Job drawing, mm, ordinate dimensions from the low corner. One solid piece. Round coordinates to 2 decimals unless told otherwise and drop trailing zeros. Loops run counter-clockwise (first coordinate to the right, second up) from the corner with the lowest first, then second, coordinate; pieces in that order, holes last.
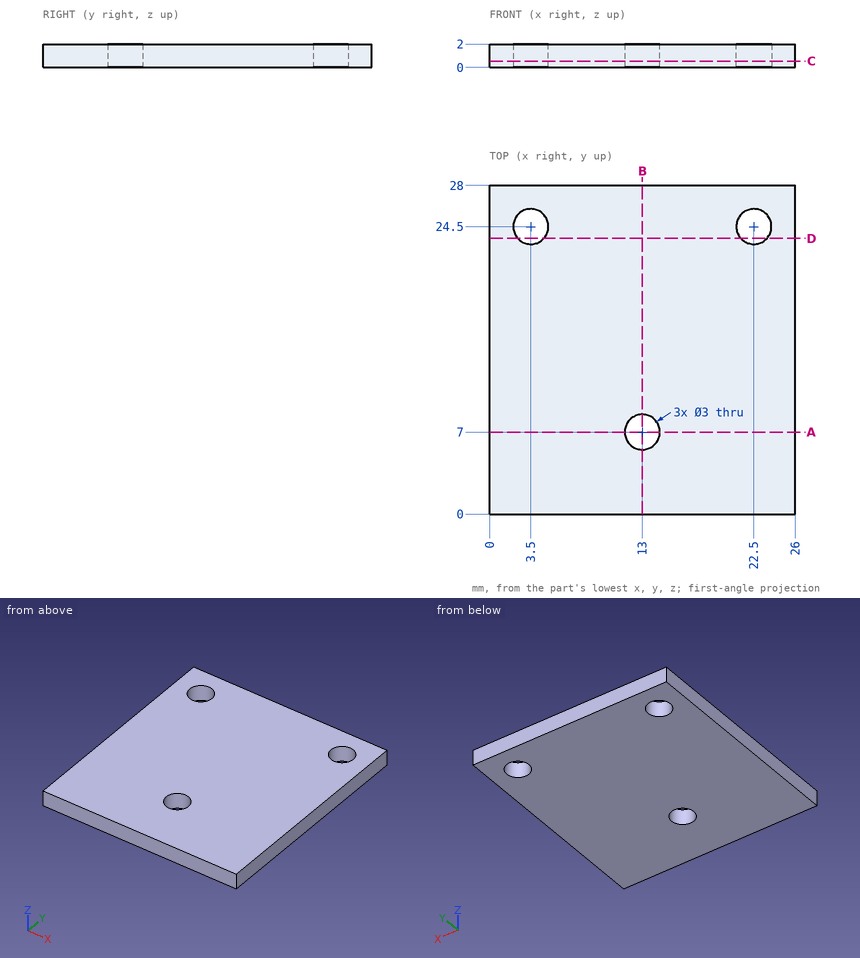
Item 1: Cut at A-A, the plane y = 7. Give the cut face in (x, z), plus the area to 3 significant figures.
Answers follow:
outline: (0, 0) - (11.5, 0) - (11.5, 2) - (0, 2) - close; (14.5, 0) - (26, 0) - (26, 2) - (14.5, 2) - close
area: 46.0 mm2
Item 2: Cut at D-D, the plane y = 23.5. Give the cut face in (x, z), plus the area to 3 significant figures.
Answers follow:
outline: (0, 0) - (2.38, 0) - (2.38, 2) - (0, 2) - close; (4.62, 0) - (21.38, 0) - (21.38, 2) - (4.62, 2) - close; (23.62, 0) - (26, 0) - (26, 2) - (23.62, 2) - close
area: 43.1 mm2
Item 3: Cut at C-C, the plane z = 0.55. Give the cut face in (x, y), plus the area to 3 significant figures.
Answers follow:
outline: (0, 0) - (26, 0) - (26, 28) - (0, 28) - close; hole circle Ø3 at (3.5, 24.5); hole circle Ø3 at (13, 7); hole circle Ø3 at (22.5, 24.5)
area: 707 mm2
Item 4: Probe line 1 (Y direction, x = 3.5, z = 0.95); line 2 (Y direction, x = 13, z = 1.2); line 3 (X direction, y = 25.75, z = 1.8). List the from-to ranges inside material, lowest first.
Answers follow:
line 1: y = 0 to 23, 26 to 28
line 2: y = 0 to 5.5, 8.5 to 28
line 3: x = 0 to 2.67, 4.33 to 21.67, 23.33 to 26
Item 5: Cut at B-B, the plane x = 13. Give the cut face in (y, z).
Answers follow:
outline: (0, 0) - (5.5, 0) - (5.5, 2) - (0, 2) - close; (8.5, 0) - (28, 0) - (28, 2) - (8.5, 2) - close
